```python
from build123d import *

# Parameters (mm, degrees)
EXTRUDE_1_DEPTH      = 30
SKETCH_2_R           = 40
EXTRUDE_2_DEPTH      = 40
CUT_EXTRUDE_1_DEPTH  = 10
CUT_EXTRUDE_2_DEPTH  = 10
SKETCH_5_R           = 26
CUT_EXTRUDE_3_DEPTH  = 269
SKETCH_6_R           = 17.5
CUT_EXTRUDE_4_DEPTH  = 269
SKETCH_7_R           = 8
CUT_EXTRUDE_5_DEPTH  = 269
SKETCH_9_W           = 30
SKETCH_9_H           = 2
CUT_EXTRUDE_8_DEPTH  = 269
SKETCH_10_R          = 2.5
CUT_EXTRUDE_9_DEPTH  = 12
SKETCH_11_R          = 3.3
CUT_EXTRUDE_10_DEPTH = 268.982


with BuildPart() as part:
    # 草图1 → 凸台-拉伸1 (new body)
    with BuildSketch(Plane.XY.offset(5)):
        with BuildLine():
            Line((2.4, -39.927935083), (201.68, -27.949554558))
            ThreePointArc((201.68, -27.949554558), (228, 0), (201.68, 27.949554558))
            Line((201.68, 27.949554558), (2.4, 39.927935083))
            ThreePointArc((2.4, 39.927935083), (-40, 0), (2.4, -39.927935083))
        make_face()
    extrude(amount=EXTRUDE_1_DEPTH)

    # 草图2 → 凸台-拉伸2 (add)
    with BuildSketch(Plane.XY):
        Circle(SKETCH_2_R)
    extrude(amount=EXTRUDE_2_DEPTH)

    # 草图3 → 切除-拉伸1 (cut)
    with BuildSketch(Plane.XY.offset(25)):
        with BuildLine():
            Line((72.2, -21.889723616), (151.4, -13.929824119))
            ThreePointArc((151.4, -13.929824119), (164, 0), (151.4, 13.929824119))
            Line((151.4, 13.929824119), (72.2, 21.889723616))
            ThreePointArc((72.2, 21.889723616), (48, 0), (72.2, -21.889723616))
        make_face()
    extrude(amount=CUT_EXTRUDE_1_DEPTH, mode=Mode.SUBTRACT)

    # 草图4 → 切除-拉伸2 (cut)
    with BuildSketch(Plane.XY.offset(5)):
        with BuildLine():
            Line((72.2, -21.889723616), (151.4, -13.929824119))
            ThreePointArc((151.4, -13.929824119), (164, 0), (151.4, 13.929824119))
            Line((151.4, 13.929824119), (72.2, 21.889723616))
            ThreePointArc((72.2, 21.889723616), (48, 0), (72.2, -21.889723616))
        make_face()
    extrude(amount=CUT_EXTRUDE_2_DEPTH, mode=Mode.SUBTRACT)

    # 草图5 → 切除-拉伸3 (cut, symmetric)
    with BuildSketch(Plane.XY):
        Circle(SKETCH_5_R)
    extrude(amount=CUT_EXTRUDE_3_DEPTH, both=True, mode=Mode.SUBTRACT)

    # 草图6 → 切除-拉伸4 (cut, symmetric)
    with BuildSketch(Plane.XY):
        with Locations((200, 0)):
            Circle(SKETCH_6_R)
    extrude(amount=CUT_EXTRUDE_4_DEPTH, both=True, mode=Mode.SUBTRACT)

    # 草图7 → 切除-拉伸5 (cut, symmetric)
    with BuildSketch(Plane.XY.offset(15)):
        with Locations((110, 0)):
            Circle(SKETCH_7_R)
    extrude(amount=CUT_EXTRUDE_5_DEPTH, both=True, mode=Mode.SUBTRACT)

    # 草图9 → 切除-拉伸8 (cut, symmetric)
    with BuildSketch(Plane.XY.offset(20)):
        with Locations((215, 0)):
            Rectangle(SKETCH_9_W, SKETCH_9_H)
    extrude(amount=CUT_EXTRUDE_8_DEPTH, both=True, mode=Mode.SUBTRACT)

    # 草图10 → 切除-拉伸9 (cut)
    with BuildSketch(Plane.XY.offset(40)):
        with Locations((28.5788, 16.5)):
            Circle(SKETCH_10_R)
        with Locations((0, 33)):
            Circle(SKETCH_10_R)
        with Locations((-28.5788, 16.5)):
            Circle(SKETCH_10_R)
        with Locations((-28.5788, -16.5)):
            Circle(SKETCH_10_R)
        with Locations((0, -33)):
            Circle(SKETCH_10_R)
        with Locations((28.5788, -16.5)):
            Circle(SKETCH_10_R)
    extrude(amount=-CUT_EXTRUDE_9_DEPTH, mode=Mode.SUBTRACT)

    # 草图11 → 切除-拉伸10 (cut, symmetric)
    with BuildSketch(Plane(origin=(0, 0, 0), x_dir=(1, 0, 0), z_dir=(0, 1, 0))):
        with Locations(Location((219, -20, 0), (0, 0, 270))):
            Circle(SKETCH_11_R)
    extrude(amount=CUT_EXTRUDE_10_DEPTH, both=True, mode=Mode.SUBTRACT)


solid = part.part
```
Geometry: final body of the model. Coordinates: model frame, mm. A direction names the side the tool comes from. Give positions to 0.01 mm unless a question says otherwise; leave off trailing zeros. Loops run counter-clockwise (first coordinate to the right, second up) from the corner with the lowest first, then second, coordinate; pieces in that order, holes last. Notation, with made-up numbers: (15, 82.25) -> (40, 82.25) arc R18 cw to (40, 114.25) -> close; hole circle Ø4 at (88, -31.75). An arc over 180 degrees is marked (long way). Use CSV: the item, a comma, the result in double quotes.
(1) Ray query, line 1 along Y through (x, z) = (0, 34.75); line 2 along Z through (x, y) = (219, -12); line 3 along X through (y, z) = (10, 20). Return the intervals inside material, ascending. Write a range as [from, to].
From the geometry:
line 1,"[-40, -35.5], [-30.5, -26], [26, 30.5], [35.5, 40]"
line 2,"[5, 16.7], [23.3, 35]"
line 3,"[-38.73, -24], [24, 185.64], [214.36, 215.7], [222.3, 226.15]"
(2) Access query for faces 4 (the face through (-29, -16, 28)), 5 (the face through (26, -8, 40)), 6 (the face through (111.246, -17.965, 9.93)). Directions: +Z, -Z, +X, -X, +Y, -Y. A direction counts if a zero-diameter tool reaches every point of the face in a straight line with its end or side. Return the directions, or none.
From the geometry:
face 4,"+Z"
face 5,"+Z, +X, -X, +Y, -Y"
face 6,"-Z"
(3) First-contact query: P1, Ø5, axis at x = 109, z = 11, coming from the -Y side; P2, Ø12, axis at x = 144.5, z = 26, coming from the -Y side; P3, Ø5.5, axis at x = 219, z = 20, coming from the -Y side; P4, Ø4, axis at x = 82, y = 20, coming from the -Z side. Flat tips, straight axial feed; report the tip coordinate or a pass-through.
From the geometry:
P1,"y = -33.67"
P2,"y = -31.75"
P3,"through"
P4,"z = 5"
(4) Cut plane B-B (z = 37.5). Output: boundary loops of the cut face in (x, y), plus the area to 3 significant figures.
From the geometry:
outline,"circle Ø80 at (0, 0); hole circle Ø5 at (-28.58, -16.5); hole circle Ø5 at (-28.58, 16.5); hole circle Ø52 at (0, 0); hole circle Ø5 at (0, -33); hole circle Ø5 at (0, 33); hole circle Ø5 at (28.58, -16.5); hole circle Ø5 at (28.58, 16.5)"
area,"2,790 mm^2"
(5) Cut plane C-C (x = 110). Output: boundary loops of the cut face in (y, z), plus the area to 3 significant figures.
From the geometry:
outline,"(-33.46, 5) -> (-18.09, 5) -> (-18.09, 15) -> (-8, 15) -> (-8, 25) -> (-18.09, 25) -> (-18.09, 35) -> (-33.46, 35) -> close; (8, 15) -> (18.09, 15) -> (18.09, 5) -> (33.46, 5) -> (33.46, 35) -> (18.09, 35) -> (18.09, 25) -> (8, 25) -> close"
area,"1,120 mm^2"
(6) Cut plane A-A (z = 11). Output: boundary loops of the cut face in (x, y), plus the area to 3 significant figures.
From the geometry:
outline,"(2.4, -39.93) -> (201.68, -27.95) arc R28 ccw to (227.98, -1) -> (217.47, -1) arc R17.5 cw (long way) to (217.47, 1) -> (227.98, 1) arc R28 ccw to (201.68, 27.95) -> (2.4, 39.93) arc R40 ccw (long way) to start; hole circle Ø52 at (0, 0); hole (72.2, -21.89) -> (151.4, -13.93) arc R14 ccw to (151.4, 13.93) -> (72.2, 21.89) arc R22 ccw (long way) to start"
area,"10,300 mm^2"
(7) Cut plane D-D (x = 8). Output: boundary loops of the cut face in (y, z), plus the area to 3 significant figures.
From the geometry:
outline,"(-39.59, 5) -> (-39.19, 5) -> (-39.19, 0) -> (-24.74, 0) -> (-24.74, 40) -> (-39.19, 40) -> (-39.19, 35) -> (-39.59, 35) -> close; (24.74, 0) -> (39.19, 0) -> (39.19, 5) -> (39.59, 5) -> (39.59, 35) -> (39.19, 35) -> (39.19, 40) -> (24.74, 40) -> close"
area,"1,180 mm^2"
(8) Pull-direction query (X, two-part tool) for faces 1 (the face through (48.006, 0.515, 29.93)), 2 (the face through (103.435, 33.855, 19.79)), 3 (the face through (223, -1, 20)); classes: released by +X, released by -X, zero draft, split by the parting line, or undercut.
From the geometry:
face 1,"undercut"
face 2,"released by +X"
face 3,"zero draft"
